from build123d import *
from build123d.topology import SkipClean

# Parameters (mm, degrees)
RESSALTO_EXTRUS_O1_DEPTH = 2
ESBO_O2_R                = 0.85
CORTE_EXTRUS_O1_DEPTH    = 17.317168872
ESBO_O4_R                = 2.5
RESSALTO_EXTRUS_O2_DEPTH = 2
CORTE_EXTRUS_O2_REACH    = 18.681
ESBO_O3_R                = 0.5
RESSALTO_EXTRUS_O3_DEPTH = 0.5


with BuildPart() as part:
    # Esbo_o1 → Ressalto-extrus_o1 (new body)
    with BuildSketch(Plane(origin=(0, 0, 0), x_dir=(1, 0, 0), z_dir=(0, 1, 0))):
        with BuildLine():
            Line((-13.5, 2.5), (13.5, 2.5))
            ThreePointArc((13.5, 2.5), (16, 0), (13.5, -2.5))
            Line((13.5, -2.5), (-13.5, -2.5))
            ThreePointArc((-13.5, -2.5), (-16, 0), (-13.5, 2.5))
        make_face()
    extrude(amount=RESSALTO_EXTRUS_O1_DEPTH)

    # Esbo_o2 → Corte-extrus_o1 (cut, through all)
    with BuildSketch(Plane(origin=(0, 2, 0), x_dir=(1, 0, 0), z_dir=(0, 1, 0))):
        with Locations(Location((-13.5, 0, 0), (0, 0, 270))):
            Circle(ESBO_O2_R)
    extrude(amount=-CORTE_EXTRUS_O1_DEPTH, mode=Mode.SUBTRACT)

    # Esbo_o4 → Ressalto-extrus_o2 (add)
    with SkipClean():  # the faces are left unmerged after this step: merging them gives an invalid solid
        with BuildSketch(Plane(origin=(0, 2, 0), x_dir=(1, 0, 0), z_dir=(0, 1, 0))):
            with Locations(Location((13.5, 0, 0), (0, 0, 270))):
                Circle(ESBO_O4_R)
        extrude(amount=RESSALTO_EXTRUS_O2_DEPTH)
    add(part.part.scale(1), mode=Mode.REPLACE)  # the faces are merged on a copy

    # Esbo_o3 → Corte-extrus_o2 (cut, up to next)
    with BuildSketch(Plane(origin=(0, 4, 0), x_dir=(1, 0, 0), z_dir=(0, 1, 0)), mode=Mode.PRIVATE) as corte_extrus_o2_sk1:
        with Locations(Location((13.5, 0, 0), (0, 0, 270))):
            Circle(ESBO_O3_R)
    corte_extrus_o2_tool1 = extrude(corte_extrus_o2_sk1.sketch, amount=-CORTE_EXTRUS_O2_REACH, mode=Mode.PRIVATE) & part.part
    add(corte_extrus_o2_tool1.solids().sort_by_distance((13.5, 4, 0))[0], mode=Mode.SUBTRACT)

    # Esbo_o5 → Ressalto-extrus_o3 (add)
    with BuildSketch(Plane(origin=(0, 2, 0), x_dir=(1, 0, 0), z_dir=(0, 1, 0))):
        Polygon((10.246141944, -1), (9.117936815, -1), (9.117936815, -0.794871795), (10.066654764, -0.794871795), (10.066654764, -0.179487179), (9.117936815, -0.179487179), (9.117936815, 0.025641026), (10.066654764, 0.025641026), (10.066654764, 0.794871795), (9.117936815, 0.794871795), (9.117936815, 1), (10.246141944, 1), align=None)
    extrude(amount=RESSALTO_EXTRUS_O3_DEPTH)


solid = part.part
CAD build for the part. Positions are in the model's coordinates, mm. Coordinates: 2 decimals unless noted, no trailing zeros. Write each loop counter-clockwise with the first axis right and the second up, starting at its lowest first coordinate (ties: lowest second). Pieces come first, ordered by that corner, then holes. Notation, with made-up numbers: M 4.25,40 L 14.25,40 A18 cw 14.25,54 Z; hole C 86,77.25 d8. An arc over 180 degrees is marked long. Answer as a JSON object with one key per item and string values. Group by question number.
1) Saw through at C-C (y = 3.3). Write the cut outline in (x, z).
2) Mould opens along Z. For faces 1 (the face through (-12.657, 1.014, -0.111)), 2 (the face through (0, 1, -2.5)), 3 (the face through (0, 1, 2.5)) say: +Z half, -Z half, draft (parallel to the pull), parting line (faces both ways), or undercut.
3) Wall check: line 1 (X direction, y = 1.15, z = 0); line 2 (Z direction, x = 9.5, y = 2.2); line 3 (Y direction, x = 2.5, z = -0.25). Give the ranges that are in metal, low to high. Write a range as from..to.
4) Saw through at D-D (z = 1.85). Write the cut outline in (x, y), plus the area to 3 significant figures.
5) Saw through at A-A (y = 0.4). Write the cut outline in (x, z), plus the area to 3 significant figures.
6) Saw through at B-B (x = 6.5). Write the cut outline in (y, z).
7) Pin check, flat tips, straight feed: pin 1 Ø0.6 at (x, y) = (10, 2.5) entering from -Z; pin 2 Ø1.5 at (y, z) = (1.5, -1.5) entering from -X; pin 3 Ø1.5 at (x, z) = (-10, 0.5) entering from +Y; pin 4 Ø2 at (x, z) = (-13.5, 0) entering from -Y. Stop position of each tip, or through.
Values follow:
{
 "1": {"outline": "C 13.5,0 d5; hole C 13.5,0 d1"},
 "2": {"face 1": "undercut", "face 2": "-Z half", "face 3": "+Z half"},
 "3": {"line 1": "x = -16..-14.35, -12.65..13, 14..16", "line 2": "z = -1..-0.79, -0.03..0.18, 0.79..1", "line 3": "y = 0..2"},
 "4": {"outline": "M -15.18,0 L 15.18,0 L 15.18,4 L 11.82,4 L 11.82,2 L -15.18,2 Z", "area": "67.5 mm2"},
 "5": {"outline": "M -13.5,-2.5 L 13.5,-2.5 A2.5 ccw 13.5,2.5 L -13.5,2.5 A2.5 ccw Z; hole C -13.5,0 d1.7; hole C 13.5,0 d1", "area": "152 mm2"},
 "6": {"outline": "M 0,-2.5 L 2,-2.5 L 2,2.5 L 0,2.5 Z"},
 "7": {"pin 1": "stops at z = -1", "pin 2": "stops at x = -15.88", "pin 3": "stops at y = 2", "pin 4": "stops at y = 0"}
}
